from build123d import *

# Parameters (mm, degrees)
F0_W      = 100
F0_H      = 30
F1_DEPTH  = 60
F2_W      = 6
F2_H      = 6
F3_DEPTH  = 2.9
F4_W      = 30
F4_H      = 30
F5_DEPTH  = 10
F7_DEPTH  = 30
F8_R      = 10
F9_DEPTH  = 5
F10_R     = 25
F11_DEPTH = 20
F12_W     = 13.155363
F12_H     = 5.945411
F13_DEPTH = 25
F14_W     = 80
F14_H     = 47.04293
F15_DEPTH = 1
F16_R     = 3
F17_DEPTH = 1
F18_W     = 6
F18_H     = 6
F19_DEPTH = 0.3
F20_R     = 22.5
F21_DEPTH = 15
F22_R     = 15
F23_DEPTH = 16.7


with BuildPart() as f1:
    # F0 (on Top) → F1 (new body)
    with BuildSketch(Plane.XY):
        with Locations((-20.653479, -13.014261)):
            Rectangle(F0_W, F0_H)
    extrude(amount=-F1_DEPTH)

    # F2 (on face) → F3 (join)
    with BuildSketch(Plane.XY):
        with Locations((-58.653479, -10.014261)):
            Rectangle(F2_W, F2_H)
    extrude(amount=F3_DEPTH)

    # F4 (on face) → F5 (join)
    with BuildSketch(Plane.XY):
        with Locations((-20.292342, -13.014261)):
            Rectangle(F4_W, F4_H)
    extrude(amount=F5_DEPTH)

    # F6 (on face) → F7 (cut)
    with BuildSketch(Plane.YZ.offset(-5.292342)):
        Polygon((-18.235888, 10), (-28.014261, 10), (-28.014261, 0), align=None)
    extrude(amount=-F7_DEPTH, mode=Mode.SUBTRACT)

    # F8 (on face) → F9 (join)
    with BuildSketch(Plane.XY):
        with Locations((14.346521, -13.014261)):
            Circle(F8_R)
    extrude(amount=F9_DEPTH)

    # F10 (on face) → F11 (join)
    with BuildSketch(Plane.XZ.offset(28.014261)):
        with Locations((-20.653479, -35)):
            Circle(F10_R)
    extrude(amount=F11_DEPTH)

    # F12 (on face) → F13 (cut)
    with BuildSketch(Plane(origin=(0, 1.985739, 0), x_dir=(-1, 0, 0), z_dir=(0, 1, 0))):
        with Locations((20.129042, 5.192092)):
            Rectangle(F12_W, F12_H)
    extrude(amount=-F13_DEPTH, mode=Mode.SUBTRACT)

    # F14 (on face) → F15 (cut)
    with BuildSketch(Plane(origin=(0, 1.985739, 0), x_dir=(-1, 0, 0), z_dir=(0, 1, 0))):
        with Locations((20.653479, -30.478535)):
            Rectangle(F14_W, F14_H)
    extrude(amount=-F15_DEPTH, mode=Mode.SUBTRACT)

    # F16 (on face) → F17 (join)
    with BuildSketch(Plane(origin=(0, 0, -60), x_dir=(1, 0, 0), z_dir=(0, 0, -1))):
        with Locations((-55.653479, 13.014261)):
            Circle(F16_R)
        with Locations((14.346521, 13.014261)):
            Circle(F16_R)
    extrude(amount=F17_DEPTH)

    # F18 (on face) → F19 (join)
    with BuildSketch(Plane.XY.offset(10)):
        with Locations((-20.406025, -6.980354)):
            Rectangle(F18_W, F18_H)
    extrude(amount=F19_DEPTH)

    # F20 (on face) → F21 (join)
    with BuildSketch(Plane.XZ.offset(48.014261)):
        with Locations((-20.653479, -35)):
            Circle(F20_R)
    extrude(amount=F21_DEPTH)

    # F22 (on face) → F23 (join)
    with BuildSketch(Plane.XZ.offset(63.014261)):
        with Locations((-20.653479, -35)):
            Circle(F22_R)
    extrude(amount=F23_DEPTH)


solid = f1.part
Could you check a few things on this model? Use its own coordinates, in mm. A direction names the side the tool comes from. Give positions to 0.01 mm unless a question says otherwise; leave off trailing zeros. Order: outer loops, then holes, each group sorted by start corner. A loop starts at its lowest first (then second) coordinate and runs counter-clockwise, first axis right, second up. Notation, with made-up numbers: (0.5, 51.5) - (4.5, 51.5) arc R8 ccw to (4.5, 63.5) - close; hole circle Ø7 at (-32, 45.5). An arc over 180 degrees is marked (long way). One line per item, written item: value. Start each with the question number.
1. If I drill on probe 1 along Z at (x, y) = (-15, -7.5); probe 2 along X at (y, z) = (-22, 4); probe 3 along Y at (x, z) = (-65, -45.5), over which ranges is the centre line in solid material (lowest first)?
2. Imagine slicing it at A-A on z = -35. List the corners of the cut face in (x, y) for me, plus the area to 3 significant figures.
3. Imagine slicing it at B-B on y = -72. List the corners of the cut face in (x, z) for me.
4. For P1, Ø1, axis at x = -41, y = -48, coming from the +Z side; P2, Ø6, axis at x = -55, z = -35, coming from the +Y side; P3, Ø5, axis at y = -9.5, z = 3.5, coming from the +X side, each with a flat end and sliding along its axis, tell me the tip position at first contact or that it passes through.
5. For faces 1 (the face through (-5.292, -10, 5)), 2 (the face through (-26.707, -10, 5)), 3 (the face through (-43, -48.014, -31)), 4 (the face through (-20, -23.014, 4)), which set-ups out of +Z, -Z, +X, -X, +Y, -Y let a thin tool reach every point of the face, with its end or its side?
6. Imagine slicing it at C-C on x = -33.5. List the corners of the cut face in (y, z) for me.
7. Thinking about a two-plate mould opening in Z: for faces 5 (the face through (-13.551, -10, 5)), 6 (the face through (4, -13, 0)), 7 (the face through (-56, -13, -61)), which applies, +Z half, -Z half, draft (parallel to the pull), parting line (faces both ways), or undercut?
8. Imagine slicing it at D-D on x = -65. List the corners of the cut face in (y, z) for me, plus the area to 3 significant figures.
Values:
1. probe 1: -60 to 2.22, 8.16 to 10
1. probe 2: -35.29 to -26.71, -13.55 to -5.29, 9.96 to 18.73
1. probe 3: -28.01 to 1.99
2. outline: (-70.65, -28.01) - (-45.65, -28.01) - (-45.65, -48.01) - (-43.15, -48.01) - (-43.15, -63.01) - (-35.65, -63.01) - (-35.65, -79.71) - (-5.65, -79.71) - (-5.65, -63.01) - (1.85, -63.01) - (1.85, -48.01) - (4.35, -48.01) - (4.35, -28.01) - (29.35, -28.01) - (29.35, 1.99) - (19.35, 1.99) - (19.35, 0.99) - (-60.65, 0.99) - (-60.65, 1.99) - (-70.65, 1.99) - close
2. area: 5,100 mm²
3. outline: circle Ø30 at (-20.65, -35)
4. P1: z = -19.8
4. P2: y = 0.99
4. P3: x = 24.29
5. face 1: +Z, +Y, -Y
5. face 2: +Y
5. face 3: -Y
5. face 4: +Z, +Y
6. outline: (-79.71, -42.74) - (-63.01, -42.74) - (-63.01, -53.47) - (-48.01, -53.47) - (-48.01, -56.45) - (-28.01, -56.45) - (-28.01, -60) - (1.99, -60) - (1.99, -54) - (0.99, -54) - (0.99, -6.96) - (1.99, -6.96) - (1.99, 10) - (-18.24, 10) - (-28.01, 0) - (-28.01, -13.55) - (-48.01, -13.55) - (-48.01, -16.53) - (-63.01, -16.53) - (-63.01, -27.26) - (-79.71, -27.26) - close
7. face 5: undercut
7. face 6: +Z half
7. face 7: -Z half
8. outline: (-28.01, -60) - (1.99, -60) - (1.99, 0) - (-28.01, 0) - close
8. area: 1,800 mm²
